For this review, take the finished solid that the model builds, in its own axes (mm). Face numbers are marked on the shaded views. A direction names the side the tool comes from. Give positions to 0.01 mm unless a question says otherwise; leave off trailing zeros. Loops run counter-clockwise (first coordinate to the right, second up) from the corner with the lowest first, then second, coordinate; pieces in that order, holes last.
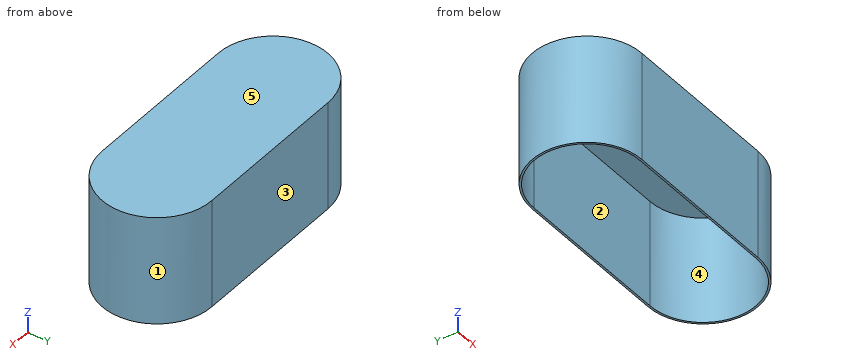
```python
from build123d import *

# Parameters (mm, degrees)
BOSS_EXTRU_2_DEPTH = 162
COQUE1_T           = 3


with BuildPart() as part:
    # Esquisse1 → Boss.-Extru.2 (new body)
    with BuildSketch(Plane.XY):
        with BuildLine():
            Line((-120, 80), (120, 80))
            ThreePointArc((120, 80), (200, 0), (120, -80))
            Line((120, -80), (-120, -80))
            ThreePointArc((-120, -80), (-200, 0), (-120, 80))
        make_face()
    extrude(amount=BOSS_EXTRU_2_DEPTH)

    # Coque1
    coque1_openings = [part.faces().sort_by_distance(p)[0] for p in [
        (0, 0, 0),
    ]]
    offset(amount=COQUE1_T, openings=coque1_openings, kind=Kind.INTERSECTION)


solid = part.part
```
Q1. For probe 1 along Y at (x, z) = (-43, 107); probe 2 along X at (y, z) = (-0.5, 148.5); probe 3 along Z at (x, y) = (156, -25), list the stretches that pass through material, from the lowest coordinate up.
Answers:
probe 1: y = -83 to -80, 80 to 83
probe 2: x = -203 to -200, 200 to 203
probe 3: z = 162 to 165
Q2. Consider section A-A on z = 152. Give the boundary of the cut face in (x, y), plus the area to 3 significant figures.
Answers:
outline: (-120, -83) - (120, -83) arc R83 ccw to (120, 83) - (-120, 83) arc R83 ccw to start; hole (-120, -80) - (120, -80) arc R80 ccw to (120, 80) - (-120, 80) arc R80 ccw to start
area: 2,980 mm2
Q3. For pin 1 Ø10 at (y, z) = (56.5, 142) entering from +X; pin 2 Ø8 at (x, y) = (-123, 61) entering from -Z; pin 3 Ø1.5 at (x, z) = (126.5, 25.5) entering from -Y, all flat-tipped, find the tip position at first contact; note any pin that passes through.
Answers:
pin 1: stops at x = 185.09
pin 2: stops at z = 162
pin 3: stops at y = -82.8
Q4. Consider section B-B on y = 0. Give the boundary of the cut face in (x, z).
Answers:
outline: (-203, 0) - (-200, 0) - (-200, 162) - (200, 162) - (200, 0) - (203, 0) - (203, 165) - (-203, 165) - close
Q5. Consider section C-C on x = 88. Give the boundary of the cut face in (y, z), plus the area to 3 significant figures.
Answers:
outline: (-83, 0) - (-80, 0) - (-80, 162) - (80, 162) - (80, 0) - (83, 0) - (83, 165) - (-83, 165) - close
area: 1,470 mm2
Q6. Mouldability with a two-part tool opening along Y and no side actions: class the marked faces 1, 2 and 3 as +Y half, -Y half, draft (parallel to the pull), parting line (faces both ways), or undercut.
Answers:
face 1: parting line
face 2: undercut
face 3: +Y half
Q7. Machinability: for the marked faces 4 and 5, which of the approach directions +Z, -Z, +X, -X, +Y, -Y give a long, thin tool a straight path to every point of the face, cutting with its end or side? Answer none if there is none.
Answers:
face 4: -Z
face 5: +Z, +X, -X, +Y, -Y
